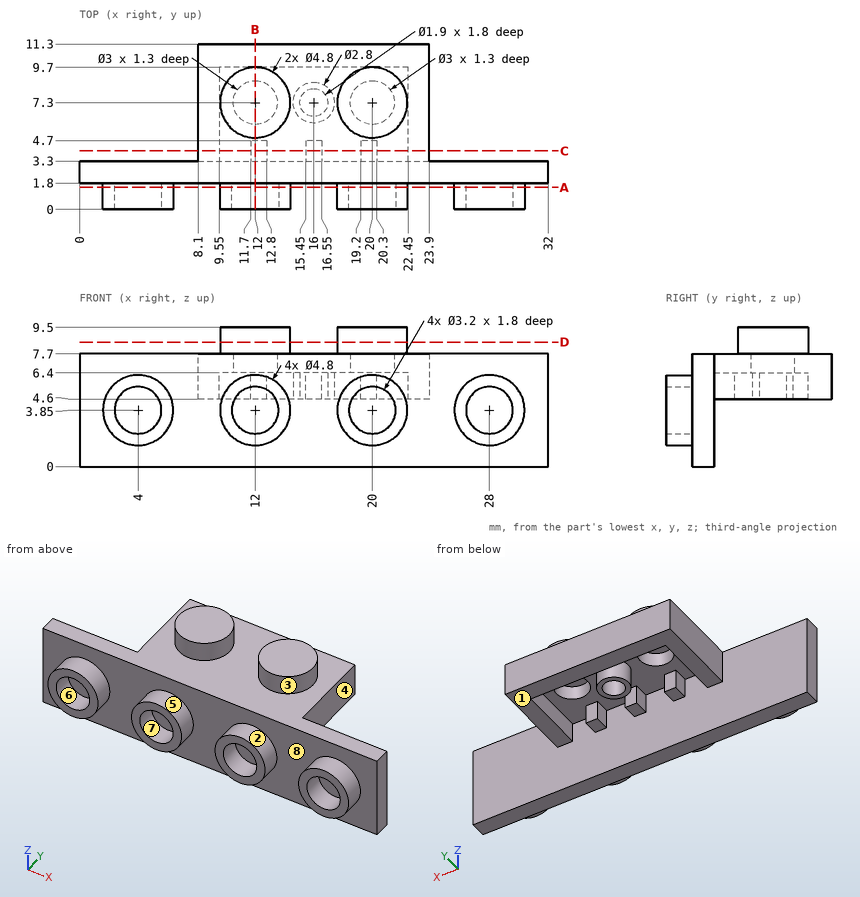
Drawing for the job (mm, zero at the part's lowest x, y, z). A direction names the side the tool comes from. Round coordinates to 2 decimals unless told otherwise and drop trailing zeros. Loops run counter-clockwise (first coordinate to the right, second up) from the corner with the lowest first, then second, coordinate; pieces in that order, holes last.
1. Mould opens along Z. For the marked faces 5, 6, 7 and 8 say: +Z half, -Z half, draft (parallel to the pull), parting line (faces both ways), or undercut.
Check values:
face 5: parting line
face 6: undercut
face 7: undercut
face 8: draft
2. Band-saw the part on B-B, the plane x = 12. List the corners of the cut face in (y, z), and give its area (3 significant figures).
Check values:
outline: (0, 1.45) - (1.8, 1.45) - (1.8, 0) - (3.3, 0) - (3.3, 4.6) - (4.7, 4.6) - (4.7, 6.4) - (5.8, 6.4) - (5.8, 7.7) - (8.8, 7.7) - (8.8, 6.4) - (9.7, 6.4) - (9.7, 4.6) - (11.3, 4.6) - (11.3, 7.7) - (9.7, 7.7) - (9.7, 9.5) - (4.9, 9.5) - (4.9, 7.7) - (1.8, 7.7) - (1.8, 6.25) - (0, 6.25) - (0, 5.45) - (1.8, 5.45) - (1.8, 2.25) - (0, 2.25) - close
area: 35.0 mm2
3. Band-saw the part on C-C, the plane y = 4. List the corners of the cut face in (x, z), and give its area (3 significant figures).
Check values:
outline: (8.1, 4.6) - (9.55, 4.6) - (9.55, 6.4) - (11.7, 6.4) - (11.7, 4.6) - (12.8, 4.6) - (12.8, 6.4) - (15.45, 6.4) - (15.45, 4.6) - (16.55, 4.6) - (16.55, 6.4) - (19.2, 6.4) - (19.2, 4.6) - (20.3, 4.6) - (20.3, 6.4) - (22.45, 6.4) - (22.45, 4.6) - (23.9, 4.6) - (23.9, 7.7) - (8.1, 7.7) - close
area: 31.7 mm2
4. Drop flat-ended pins along their axis: P1, Ø2.5, axis at x = 20.5, y = 7, coming from the -Z side; P2, Ø1.2, axis at x = 15.5, y = 4, coming from the -Z side; P3, Ø3, axis at x = 7.5, z = 7, coming from the +Y side; P4, Ø1, axis at x = 28, z = 3, coming from the -Y side. Give the stop position or say it passes through.
Check values:
P1: stops at z = 6.4
P2: stops at z = 4.6
P3: stops at y = 11.3
P4: stops at y = 1.8
5. Band-saw the part on D-D, the plane z = 8.5. List the corners of the cut face in (x, y), and give its area (3 significant figures).
Check values:
outline: circle Ø4.8 at (12, 7.3); circle Ø4.8 at (20, 7.3)
area: 36.2 mm2
6. Wall check: probe 1 along X at (y, z) = (7.3, 7.3); probe 2 along X at (y, z) = (7.25, 6); probe 3 along Z at (x, y) = (12, 1.25). Give the ranges that are in metal, low to high.
Check values:
probe 1: x = 8.1 to 10.5, 13.5 to 18.5, 21.5 to 23.9
probe 2: x = 8.1 to 9.55, 14.6 to 15.05, 16.95 to 17.4, 22.45 to 23.9
probe 3: z = 1.45 to 2.25, 5.45 to 6.25
7. Band-saw the part on A-A, the plane y = 1.5. List the corners of the cut face in (x, z).
Check values:
outline: circle Ø4.8 at (4, 3.85); circle Ø4.8 at (12, 3.85); circle Ø4.8 at (20, 3.85); circle Ø4.8 at (28, 3.85); hole circle Ø3.2 at (4, 3.85); hole circle Ø3.2 at (12, 3.85); hole circle Ø3.2 at (20, 3.85); hole circle Ø3.2 at (28, 3.85)
8. Tool access for the marked faces 1, 2, 3 and 4: list every direction of +Z, -Z, +X, -X, +Y, -Y with a clear straight run to the whole face (end or side of a thin tool).
Check values:
face 1: -Z, +X, -X, +Y
face 2: -Y
face 3: +Z
face 4: +Z, -Z, +X, +Y
